Here's how the part is built. I have some questions about the finished solid (model axes, mm). A direction names the side the tool comes from. Round coordinates to 2 decimals unless told otherwise and drop trailing zeros. Write each loop counter-clockwise with the first axis right and the second up, starting at its lowest first coordinate (ties: lowest second). Pieces come first, ordered by that corner, then holes. Notation, with made-up numbers: (43.5, 38) -> (59.5, 38) arc R32 cw to (59.5, 66) -> close; hole circle Ø7 at (50.25, 72). An arc over 180 degrees is marked (long way). Put each result on its own line as item: value. Start each with the question number.
1) I want a section at C-C, the plane y = 4.25. List the corners of the cut face in (x, z) for me.
2) If I drill on line 1 along X through (y, z) = (9.25, 8.5); line 2 along Z through (x, y) = (-13, 1.25); line 3 along Y through (x, z) = (-2, 0.75), over which ranges is the centre line in solid material (lowest first)? Write a range as [from, to].
3) I want a section at A-A, the plane z = 6.75. List the corners of the cut face in (x, y) for me, then the cut area to 3 significant figures.
4) We'd pull the mould along X, two halves only. Please class faces 6 (the cylindrical face through (-13.52, 8.82, 2.63)), 7 (the flat face through (-2.524, 7.379, 2.129)), 8 (the flat face through (-1.3, 4.572, 0.7)): released by +X, released by -X, zero draft, split by the parting line, or undercut.
5) I want a section at B-B, the plane y = 11.25. List the corners of the cut face in (x, z) for me.
6) Will these pins go through, and if not, where does the flat tip stop? P1, Ø0.6, axis at y = 0.5, z = 3, coming from the -X side; P2, Ø3, axis at y = 6, z = 1, coming from the +X side; P3, Ø0.8, axis at x = -6, z = 3, coming from the -Y side; P4, Ø1.3, axis at y = 3.5, z = 0.5, coming from the +X side.
7) I want a section at D-D, the plane x = -13. List the corners of the cut face in (y, z) for me.
8) Which directions (+Z, -Z, +X, -X, +Y, -Y) give clear straight access to the entire face, cutting with the end or side of a thin tool? Please do faces 1 (the flat face through (-6, 6.57, 3)), 2 (the flat face through (-9, 11.938, 5)), 3 (the cylindrical face through (-10.859, 8.876, 2.63)), 4 (the flat face through (-5.08, 6, 8)), 5 (the flat face through (-2.159, 4, 1)).
from build123d import *

# Parameters (mm, degrees)
EXTRUDE1_DEPTH          = 4.7752
EXTRUDE2_DEPTH          = 12.938
SKETCH33_W              = 2.286
SKETCH33_H              = 5.588
EXTRUDE30_DEPTH         = 10.668
EXTRUDE3_DEPTH          = 3.0988
EXTRUDE6_DEPTH          = 3.0988
EXTRUDE7_DEPTH          = 3.0988
SKETCH23_W              = 3.0988
SKETCH23_H              = 1.133450424
EXTRUDE20_DEPTH         = 2.54
EXTRUDE16_DEPTH         = 3.0988
FILLET1_R               = 0.762
EXTRUDE21_DEPTH         = 3.0988
FILLET2_R               = 0.762
EXTRUDE28_DEPTH         = 8.0612
EXTRUDE29_REACH         = 9.061
FILLET3_R               = 0.762
FILLET4_R               = 0.508
FILLET5_R               = 0.508
FILLET6_R               = 0.508
SKETCH35_R              = 1.016
EXTRUDE32_DEPTH         = 8.0612
BOSS_EXTRUDE1_DEPTH     = 5.334
BOSS_EXTRUDE2_DEPTH     = 5.334
SKETCH39_W              = 7.76878052
SKETCH39_H              = 12.502157979
CUT_EXTRUDE1_DEPTH      = 15.8590001
SKETCH40_W              = 5.041406472
SKETCH40_H              = 6.35
SKETCH40_W_2            = 0.038593528
SKETCH40_H_2            = 4.318
CUT_EXTRUDE2_DEPTH      = 1.0000001
CUT_EXTRUDE2_DEPTH_BACK = 12.9380001


with BuildPart() as part:
    # Sketch1 → Extrude1 (new body)
    with BuildSketch(Plane.XY):
        Polygon((-14.859, 11.938), (0, 11.938), (0, 4.572), (-3.175, 4.572), (-3.175, 0), (-14.859, 0), align=None)
    extrude(amount=-EXTRUDE1_DEPTH)

    # Sketch2 → Extrude2 (cut, through all)
    with BuildSketch(Plane(origin=(0, 11.938, 0), x_dir=(1, 0, 0), z_dir=(0, 1, 0))):
        Polygon((0, 0.5842), (-4.191, 4.7752), (0, 4.7752), align=None)
    extrude(amount=-EXTRUDE2_DEPTH, mode=Mode.SUBTRACT)

    # Sketch33 → Extrude30 (add)
    with BuildSketch(Plane.ZY.offset(14.859)):
        with Locations((-5.9182, 9.144)):
            Rectangle(SKETCH33_W, SKETCH33_H)
    extrude(amount=-EXTRUDE30_DEPTH)

    # Sketch5 → Extrude3 (cut)
    with BuildSketch(Plane.XY):
        with BuildLine():
            Line((-14.859, 8.121520088), (-14.859, 0))
            Line((-14.859, 0), (-8.374207602, 0))
            ThreePointArc((-8.374207602, 0), (-5.258197931, 4.182323512), (-8.261178378, 8.44652973))
            ThreePointArc((-8.261178378, 8.44652973), (-10.099280239, 8.911418564), (-11.9888, 9.0678))
            ThreePointArc((-11.9888, 9.0678), (-13.499883528, 8.825128765), (-14.859, 8.121520088))
        make_face()
    extrude(amount=-EXTRUDE3_DEPTH, mode=Mode.SUBTRACT)

    # Sketch8 → Extrude6 (add)
    with BuildSketch(Plane.XY):
        with BuildLine():
            Line((-5.916117419, 6.569687461), (-7.995771884, 6.569687461))
            ThreePointArc((-7.995771884, 6.569687461), (-8.381805974, 7.063274265), (-8.837117419, 7.493787609))
            Line((-8.837117419, 7.493787609), (-8.837117419, 8.601687461))
            ThreePointArc((-8.837117419, 8.601687461), (-7.16441835, 7.890723622), (-5.916117419, 6.569687461))
        make_face()
    extrude(amount=-EXTRUDE6_DEPTH)

    # Sketch9 → Extrude7 (add)
    with BuildSketch(Plane.XY):
        with BuildLine():
            Line((-5.916117419, 1.913912539), (-7.995771884, 1.913912539))
            ThreePointArc((-7.995771884, 1.913912539), (-8.381805974, 1.420325735), (-8.837117419, 0.989812391))
            Line((-8.837117419, 0.989812391), (-8.837117419, 0))
            Line((-8.837117419, 0), (-8.374207602, 0))
            ThreePointArc((-8.374207602, 0), (-6.971998867, 0.734557469), (-5.916117419, 1.913912539))
        make_face()
    extrude(amount=-EXTRUDE7_DEPTH)

    # Sketch23 → Extrude20 (add)
    with BuildSketch(Plane.ZY.offset(8.837117419)):
        with Locations((-1.5494, 8.060512821)):
            Rectangle(SKETCH23_W, SKETCH23_H)
    extrude(amount=-EXTRUDE20_DEPTH)

    # Sketch18 → Extrude16 (cut)
    with BuildSketch(Plane.XY):
        with BuildLine():
            Line((-4.903581733, 6.569687461), (-5.916117419, 6.569687461))
            ThreePointArc((-5.916117419, 6.569687461), (-5.2578, 4.2418), (-5.916117419, 1.913912539))
            Line((-5.916117419, 1.913912539), (-4.903581733, 1.913912539))
            ThreePointArc((-4.903581733, 1.913912539), (-4.3688, 4.2418), (-4.903581733, 6.569687461))
        make_face()
    extrude(amount=-EXTRUDE16_DEPTH, mode=Mode.SUBTRACT)

    # Fillet1
    fillet1_edges = [part.edges().sort_by_distance(p)[0] for p in [
        (0, 8.255, -0.5842),
    ]]
    fillet(fillet1_edges, radius=FILLET1_R)

    # Sketch24 → Extrude21 (add)
    with BuildSketch(Plane.XY):
        with BuildLine():
            Line((-8.837117419, 7.493787609), (-9.830149409, 8.301066631))
            ThreePointArc((-9.830149409, 8.301066631), (-10.843412246, 8.870424655), (-11.9888, 9.0678))
            Line((-11.9888, 9.0678), (-8.837117419, 9.0678))
            Line((-8.837117419, 9.0678), (-8.837117419, 7.493787609))
        make_face()
    extrude(amount=-EXTRUDE21_DEPTH)

    # Fillet2
    fillet2_edges = [part.edges().sort_by_distance(p)[0] for p in [
        (-14.859, 0, -3.937),
    ]]
    fillet(fillet2_edges, radius=FILLET2_R)

    # Sketch31 → Extrude28 (cut, through all)
    with BuildSketch(Plane.XY):
        Polygon((-3.175, 1.499352844), (-4.224858164, 0), (-3.175, 0), align=None)
    extrude(amount=-EXTRUDE28_DEPTH, mode=Mode.SUBTRACT)

    # Extrude29: up to this face of the body (flat: up to its plane)
    extrude29_end = Plane(part.part.faces().sort_by_distance((-2.383005057, 7.601249614, -2.967205057))[0])
    # Sketch32 → Extrude29 (add, up to the picked face)
    with BuildSketch(Plane.XY, mode=Mode.PRIVATE) as extrude29_sk1:
        Polygon((-3.175, 1.499352844), (-2.159, 2.950351219), (-2.159, 4.572), (-3.175, 4.572), align=None)
    extrude29_tool1 = split(extrude(extrude29_sk1.sketch, amount=-EXTRUDE29_REACH, mode=Mode.PRIVATE), bisect_by=extrude29_end, keep=Keep.BOTH, mode=Mode.PRIVATE)
    add(extrude29_tool1.solids().sort_by_distance((-2.719341, 3.361051, 0))[0])

    # Fillet3
    fillet3_edges = [part.edges().sort_by_distance(p)[0] for p in [
        (-4.224858164, 0, -2.3876),
    ]]
    fillet(fillet3_edges, radius=FILLET3_R)

    # Fillet4
    fillet4_edges = [part.edges().sort_by_distance(p)[0] for p in [
        (-3.078168199, 1.637642987, 0),
        (-4.269677813, 0.086097745, 0),
        (-6.729323838, 0, 0),
    ]]
    fillet(fillet4_edges, radius=FILLET4_R)

    # Fillet5
    fillet5_edges = [part.edges().sort_by_distance(p)[0] for p in [
        (-9.525, 11.938, -7.0612),
        (-9.525, 6.35, -7.0612),
        (-7.4295, 11.938, 0),
        (-14.859, 11.938, -3.5306),
    ]]
    fillet(fillet5_edges, radius=FILLET5_R)

    # Fillet6
    fillet6_edges = [part.edges().sort_by_distance(p)[0] for p in [
        (-7.995771884, 6.569687461, -1.5494),
        (-8.837117419, 0.989812391, -1.5494),
        (-7.995771884, 1.913912539, -1.5494),
    ]]
    fillet(fillet6_edges, radius=FILLET6_R)

    # Sketch35 → Extrude32 (cut, through all)
    with BuildSketch(Plane.XY):
        with Locations((-6.731, 8.763)):
            Circle(SKETCH35_R)
    extrude(amount=-EXTRUDE32_DEPTH, mode=Mode.SUBTRACT)

    # Sketch37 → Boss-Extrude1 (add)
    with BuildSketch(Plane.XY):
        with BuildLine():
            Line((-8.837117419, 0.508), (-8.837117419, 0))
            Line((-8.837117419, 0), (-4.621530256, 0))
            ThreePointArc((-4.621530256, 0), (-4.269677813, 0.086097745), (-3.997336399, 0.324934756))
            Line((-3.997336399, 0.324934756), (-2.159, 2.950351219))
            Line((-2.159, 2.950351219), (-2.159, 3.836022191))
            Line((-2.159, 3.836022191), (-2.159, 4.572))
            Line((-2.159, 4.572), (0, 4.572))
            Line((0, 4.572), (0, 11.43))
            Line((0, 11.43), (0, 11.878036743))
            add(Edge.make_bspline(
                [(0, 11.878036743), (0, 11.918150491), (-0.011858122, 11.938), (-0.038593528, 11.938)],
                knots=[0, 0, 0, 0, 1, 1, 1, 1], degree=3))
            Line((-0.038593528, 11.938), (-14.351, 11.938))
            ThreePointArc((-14.351, 11.938), (-14.710210245, 11.789210245), (-14.859, 11.43))
            Line((-14.859, 11.43), (-14.859, 8.121520088))
            ThreePointArc((-14.859, 8.121520088), (-13.499883528, 8.825128765), (-11.9888, 9.0678))
            ThreePointArc((-11.9888, 9.0678), (-10.843412246, 8.870424655), (-9.830149409, 8.301066631))
            Line((-9.830149409, 8.301066631), (-8.837117419, 7.493787609))
            ThreePointArc((-8.837117419, 7.493787609), (-8.466362979, 7.153440508), (-8.139079327, 6.771105032))
            ThreePointArc((-8.139079327, 6.771105032), (-7.96020818, 6.622820517), (-7.734022276, 6.569687461))
            Line((-7.734022276, 6.569687461), (-4.903581733, 6.569687461))
            ThreePointArc((-4.903581733, 6.569687461), (-4.3688, 4.2418), (-4.903581733, 1.913912539))
            Line((-4.903581733, 1.913912539), (-7.734022276, 1.913912539))
            ThreePointArc((-7.734022276, 1.913912539), (-7.96020818, 1.860779483), (-8.139079327, 1.712494968))
            ThreePointArc((-8.139079327, 1.712494968), (-8.390857142, 1.410416216), (-8.66983986, 1.133265926))
            ThreePointArc((-8.66983986, 1.133265926), (-8.793418506, 0.962601304), (-8.837117419, 0.756473917))
            Line((-8.837117419, 0.756473917), (-8.837117419, 0.508))
        make_face()
    extrude(amount=BOSS_EXTRUDE1_DEPTH)

    # Sketch38 → Boss-Extrude2 (add)
    with BuildSketch(Plane.XY.offset(5.334)):
        with BuildLine():
            Line((-0.038593528, 11.938), (-14.351, 11.938))
            ThreePointArc((-14.351, 11.938), (-14.710210245, 11.789210245), (-14.859, 11.43))
            Line((-14.859, 11.43), (-14.859, 0.762))
            ThreePointArc((-14.859, 0.762), (-14.635815367, 0.223184633), (-14.097, 0))
            Line((-14.097, 0), (-4.621530256, 0))
            ThreePointArc((-4.621530256, 0), (-4.269677813, 0.086097745), (-3.997336399, 0.324934756))
            Line((-3.997336399, 0.324934756), (-2.159, 2.950351219))
            Line((-2.159, 2.950351219), (-2.159, 4.572))
            Line((-2.159, 4.572), (0, 4.572))
            Line((0, 4.572), (0, 11.878036743))
            add(Edge.make_bspline(
                [(0, 11.878036743), (0, 11.918150491), (-0.011858122, 11.938), (-0.038593528, 11.938)],
                knots=[0, 0, 0, 0, 1, 1, 1, 1], degree=3))
        make_face()
    extrude(amount=BOSS_EXTRUDE2_DEPTH)

    # Sketch39 → Cut-Extrude1 (cut, through all)
    with BuildSketch(Plane.ZY.offset(14.859)):
        with Locations((-3.88439026, 6.25107899)):
            Rectangle(SKETCH39_W, SKETCH39_H)
    extrude(amount=-CUT_EXTRUDE1_DEPTH, mode=Mode.SUBTRACT)

    # Sketch40 → Cut-Extrude2 (cut, two sides)
    with BuildSketch(Plane(origin=(0, 11.938, 0), x_dir=(1, 0, 0), z_dir=(0, 1, 0))) as cut_extrude2_sk:
        Polygon((-0.038593528, 0), (-5.08, -4.318), (-0.038593528, -4.318), align=None)
        with Locations((-2.559296764, -7.493)):
            Rectangle(SKETCH40_W, SKETCH40_H)
        with Locations((-0.019296764, -2.159)):
            Rectangle(SKETCH40_W_2, SKETCH40_H_2)
        with Locations((-0.019296764, -7.493)):
            Rectangle(SKETCH40_W_2, SKETCH40_H)
    extrude(amount=CUT_EXTRUDE2_DEPTH, mode=Mode.SUBTRACT)
    extrude(cut_extrude2_sk.sketch, amount=-CUT_EXTRUDE2_DEPTH_BACK, mode=Mode.SUBTRACT)


solid = part.part
Findings:
1. outline: (-14.86, 5.33) -> (-5.08, 5.33) -> (-5.08, 10.67) -> (-14.86, 10.67) -> close; (-4.37, 0) -> (-2.16, 0) -> (-2.16, 1.82) -> (-4.37, 3.71) -> close
2. line 1: x = [-14.86, -5.08]
2. line 2: z = [5.33, 10.67]
2. line 3: y = [4.57, 11.94]
3. outline: (-14.86, 0.76) arc R0.76 ccw to (-14.1, 0) -> (-5.08, 0) -> (-5.08, 11.94) -> (-14.35, 11.94) arc R0.51 ccw to (-14.86, 11.43) -> close
3. area: 117 mm2
4. face 6: undercut
4. face 7: released by +X
4. face 8: zero draft
5. outline: (-14.86, 0) -> (-0.04, 0) -> (-5.08, 4.32) -> (-5.08, 10.67) -> (-14.86, 10.67) -> close
6. P1: stops at x = -8.84
6. P2: stops at x = -0.04
6. P3: stops at y = 0
6. P4: stops at x = -2.16
7. outline: (0, 5.33) -> (8.96, 5.33) -> (8.96, 0) -> (11.94, 0) -> (11.94, 10.67) -> (0, 10.67) -> close
8. face 1: -Z, -X
8. face 2: +Z, -Z, +X, -X, +Y
8. face 3: -Z, -Y
8. face 4: +Z, +X, +Y, -Y
8. face 5: +Z, -Z, +X, -Y
